Here's how the part is built. I have some questions about the finished solid (model axes, mm). A direction names the side the tool comes from. Coordinates: 2 decimals unless noted, no trailing zeros. Order: outer loops, then holes, each group sorted by start corner. A loop starts at its lowest first (then second) coordinate and runs counter-clockwise, first axis right, second up. Notation, with made-up numbers: M 36.25,41.5 L 93.25,41.5 A21 ccw 93.25,61.5 Z; hole C 11,18.5 d9. An arc over 180 degrees is marked long. One line per question, with ' | ' between items. Start each with the question number.
```python
from build123d import *

# Parameters (mm, degrees)
SKETCH1_W           = 100
SKETCH1_H           = 200
SKETCH1_W_2         = 67
SKETCH1_H_2         = 110
BOSS_EXTRUDE1_DEPTH = 2
SKETCH2_W           = 100
SKETCH2_H           = 200
SKETCH2_W_2         = 94
SKETCH2_H_2         = 194
BOSS_EXTRUDE2_DEPTH = 16.4
SKETCH3_R           = 1.15
BOSS_EXTRUDE3_DEPTH = 2
BOSS_EXTRUDE4_DEPTH = 25
SKETCH8_W           = 100
SKETCH8_H           = 110
BOSS_EXTRUDE5_DEPTH = 3
SKETCH9_W           = 11
SKETCH9_H           = 13
CUT_EXTRUDE2_DEPTH  = 36
SKETCH10_W          = 7
SKETCH10_H          = 3
CUT_EXTRUDE3_DEPTH  = 10
SKETCH11_W          = 3
SKETCH11_H          = 7
CUT_EXTRUDE4_DEPTH  = 10
SKETCH12_W          = 100
SKETCH12_H          = 17.4
CUT_EXTRUDE5_DEPTH  = 3
SKETCH13_W          = 146.237469439
SKETCH13_H          = 217.9364229
CUT_EXTRUDE6_DEPTH  = 57
SKETCH14_R          = 2
CUT_EXTRUDE7_DEPTH  = 57
SKETCH15_W          = 2
SKETCH15_H          = 10
SKETCH15_W_2        = 10
SKETCH15_H_2        = 2
BOSS_EXTRUDE6_DEPTH = 5
SKETCH16_W          = 10
SKETCH16_H          = 1.7
BOSS_EXTRUDE7_DEPTH = 2
SKETCH17_W          = 10
SKETCH17_H          = 1.7
BOSS_EXTRUDE8_DEPTH = 2


with BuildPart() as part:
    # Sketch1 → Boss-Extrude1 (new body)
    with BuildSketch(Plane(origin=(0, 0, 0), x_dir=(1, 0, 0), z_dir=(0, 1, 0))):
        Rectangle(SKETCH1_W, SKETCH1_H)
        with Locations((0, 35)):
            Rectangle(SKETCH1_W_2, SKETCH1_H_2, mode=Mode.SUBTRACT)
    extrude(amount=BOSS_EXTRUDE1_DEPTH)

    # Sketch2 → Boss-Extrude2 (add)
    with BuildSketch(Plane.XZ):
        Rectangle(SKETCH2_W, SKETCH2_H)
        Rectangle(SKETCH2_W_2, SKETCH2_H_2, mode=Mode.SUBTRACT)
    extrude(amount=BOSS_EXTRUDE2_DEPTH)

    # Sketch3 → Boss-Extrude3 (add)
    with BuildSketch(Plane.XZ.offset(16.4)):
        Polygon((-50, 100), (50, 100), (50, 10), (50, -9), (30, -9), (30, 1), (35, 1), (35, 10), (35, 80), (-35, 80), (-35, 10), (-35, 1), (-30, 1), (-30, -9), (-50, -9), (-50, 10), align=None)
        with Locations(Location((-35, 85, 0), (0, 0, 270))):
            Circle(SKETCH3_R, mode=Mode.SUBTRACT)
        with Locations(Location((35, 85, 0), (0, 0, 270))):
            Circle(SKETCH3_R, mode=Mode.SUBTRACT)
        with Locations(Location((-35, -4, 0), (0, 0, 270))):
            Circle(SKETCH3_R, mode=Mode.SUBTRACT)
        with Locations(Location((35, -4, 0), (0, 0, 270))):
            Circle(SKETCH3_R, mode=Mode.SUBTRACT)
    extrude(amount=BOSS_EXTRUDE3_DEPTH)

    # Sketch5 → Boss-Extrude4 (add)
    with BuildSketch(Plane.XZ.offset(16.4)):
        Polygon((-50, -100), (50, -100), (50, -97), (50, 10), (47, 10), (47, -97), (-47, -97), (-47, 10), (-50, 10), (-50, -97), align=None)
    extrude(amount=BOSS_EXTRUDE4_DEPTH)

    # Sketch8 → Boss-Extrude5 (add)
    with BuildSketch(Plane.XZ.offset(41.4)):
        with Locations((0, -45)):
            Rectangle(SKETCH8_W, SKETCH8_H)
    extrude(amount=BOSS_EXTRUDE5_DEPTH)

    # Sketch9 → Cut-Extrude2 (cut)
    with BuildSketch(Plane(origin=(0, -16.4, 0), x_dir=(1, 0, 0), z_dir=(0, 1, 0))):
        with Locations((-28.65, -74.5)):
            Rectangle(SKETCH9_W, SKETCH9_H)
        with Locations((-0.71, -74.5)):
            Rectangle(SKETCH9_W, SKETCH9_H)
        with Locations((24.69, -74.5)):
            Rectangle(SKETCH9_W, SKETCH9_H)
        with Locations((-28.65, -49.1)):
            Rectangle(SKETCH9_W, SKETCH9_H)
        with Locations((-0.71, -49.1)):
            Rectangle(SKETCH9_W, SKETCH9_H)
        with Locations((24.69, -49.1)):
            Rectangle(SKETCH9_W, SKETCH9_H)
    extrude(amount=CUT_EXTRUDE2_DEPTH, mode=Mode.SUBTRACT)

    # Sketch10 → Cut-Extrude3 (cut)
    with BuildSketch(Plane.XZ.offset(44.4)):
        with Locations((-39.5, 5)):
            Rectangle(SKETCH10_W, SKETCH10_H)
        with Locations((39.5, 5)):
            Rectangle(SKETCH10_W, SKETCH10_H)
    extrude(amount=-CUT_EXTRUDE3_DEPTH, mode=Mode.SUBTRACT)

    # Sketch11 → Cut-Extrude4 (cut)
    with BuildSketch(Plane.XZ.offset(18.4)):
        with Locations((-45, 91.5)):
            Rectangle(SKETCH11_W, SKETCH11_H)
        with Locations((45, 91.5)):
            Rectangle(SKETCH11_W, SKETCH11_H)
    extrude(amount=-CUT_EXTRUDE4_DEPTH, mode=Mode.SUBTRACT)

    # Sketch12 → Cut-Extrude5 (cut)
    with BuildSketch(Plane.XY.offset(100)):
        with Locations((0, -9.7)):
            Rectangle(SKETCH12_W, SKETCH12_H)
    extrude(amount=-CUT_EXTRUDE5_DEPTH, mode=Mode.SUBTRACT)

    # Sketch13 → Cut-Extrude6 (cut)
    with BuildSketch(Plane.XZ):
        with Locations((11.358250054, -1.301466152)):
            Rectangle(SKETCH13_W, SKETCH13_H)
    extrude(amount=CUT_EXTRUDE6_DEPTH, mode=Mode.SUBTRACT)

    # Sketch14 → Cut-Extrude7 (cut)
    with BuildSketch(Plane(origin=(0, 2, 0), x_dir=(1, 0, 0), z_dir=(0, 1, 0))):
        with Locations(Location((-41, -91, 0), (0, 0, 270))):
            Circle(SKETCH14_R)
        with Locations(Location((41, -91, 0), (0, 0, 270))):
            Circle(SKETCH14_R)
        with Locations(Location((41, -32.5, 0), (0, 0, 270))):
            Circle(SKETCH14_R)
        with Locations(Location((-41, -32.5, 0), (0, 0, 270))):
            Circle(SKETCH14_R)
        with Locations(Location((-41, 91, 0), (0, 0, 270))):
            Circle(SKETCH14_R)
        with Locations(Location((41, 91, 0), (0, 0, 270))):
            Circle(SKETCH14_R)
    extrude(amount=-CUT_EXTRUDE7_DEPTH, mode=Mode.SUBTRACT)

    # Sketch15 → Boss-Extrude6 (add)
    with BuildSketch(Plane.XZ):
        with Locations((-36.8, 3.147463841)):
            Rectangle(SKETCH15_W, SKETCH15_H)
        with Locations((-36.8, -72.12250392)):
            Rectangle(SKETCH15_W, SKETCH15_H)
        with Locations((40.8, 5)):
            Rectangle(SKETCH15_W, SKETCH15_H)
        with Locations((40.8, -72.12250392)):
            Rectangle(SKETCH15_W, SKETCH15_H)
        with Locations((-1.11415266, -96)):
            Rectangle(SKETCH15_W_2, SKETCH15_H_2)
        with Locations((-1.11415266, 27)):
            Rectangle(SKETCH15_W_2, SKETCH15_H_2)
    extrude(amount=BOSS_EXTRUDE6_DEPTH)

    # Sketch16 → Boss-Extrude7 (add)
    with BuildSketch(Plane(origin=(-35.8, 0, 0), x_dir=(0, 0, -1), z_dir=(1, 0, 0))):
        with Locations((-3.147463841, -4.15)):
            Rectangle(SKETCH16_W, SKETCH16_H)
        with Locations((72.12250392, -4.15)):
            Rectangle(SKETCH16_W, SKETCH16_H)
    extrude(amount=BOSS_EXTRUDE7_DEPTH)

    # Sketch17 → Boss-Extrude8 (add)
    with BuildSketch(Plane.ZY.offset(-39.8)):
        with Locations((5, -4.15)):
            Rectangle(SKETCH17_W, SKETCH17_H)
        with Locations((-72.12250392, -4.15)):
            Rectangle(SKETCH17_W, SKETCH17_H)
    extrude(amount=BOSS_EXTRUDE8_DEPTH)


solid = part.part
```
1. Which directions (+Z, -Z, +X, -X, +Y, -Y) give clear straight access to the entire face, cutting with the end or side of a thin tool? Please do faces 1 (the face through (40, -3, -67.123)), 2 (the face through (41.8, -2, 5)), 3 (the face through (-36, -3, -77.123)).
2. Will these pins go through, and if not, where does the flat tip stop? pin 1 (4 mm diameter, centred on y = -3.5, z = -71, fed in from +X); pin 2 (2.5 mm diameter, centred on y = -2.5, z = 7.5, fed in from -X); pin 3 (1.6 mm diameter, centred on y = -2.5, z = -96.5, fed in from +X).
3. We'd pull the mould along Z, two halves only. Please class faces 4 (the face through (-36, -3, -1.853)), 5 (the face through (-37.8, -2, 3)), 6 (the face through (-1, -2, 28)): released by +Z, released by -Z, zero draft, split by the parting line, or undercut.
4. Imagine slicing it at D-D (y = -2). List the corners of the cut face in (x, z) for me, then the cut area to 3 significant figures.
5. Imagine slicing it at C-C (z = 91). List the corners of the cut face in (x, y) for me, then the cut area to 3 significant figures.
6. Imagine slicing it at B-B (z = 3.5). List the corners of the cut face in (x, y) for me.
7. Imagine slicing it at A-A (x = -41). List the corners of the cut face in (y, z) for me.
8. I need wall thicknesses on line 1 (X direction, y = 1.05, z = 91); line 2 (Z direction, x = -6, y = 1.25); line 3 (Z direction, x = -16, y = 1.25). Which ranges of each line are inside material? Lowest first, please.
Entries:
1) face 1: +X, -X, -Y | face 2: +Z, -Z, +X, -Y | face 3: -Z, +X, -X, -Y
2) pin 1: x = 41.8 | pin 2: x = -37.8 | pin 3: x = 3.89
3) face 4: undercut | face 5: zero draft | face 6: released by +Z
4) outline: M -37.8,-77.12 L -35.8,-77.12 L -35.8,-67.12 L -37.8,-67.12 Z; M -37.8,-1.85 L -35.8,-1.85 L -35.8,8.15 L -37.8,8.15 Z; M -6.11,-97 L 3.89,-97 L 3.89,-95 L -6.11,-95 Z; M -6.11,26 L 3.89,26 L 3.89,28 L -6.11,28 Z; M 39.8,-77.12 L 41.8,-77.12 L 41.8,-67.12 L 39.8,-67.12 Z; M 39.8,0 L 41.8,0 L 41.8,10 L 39.8,10 Z | area: 120 mm²
5) outline: M -50,0 L -43,0 L -43,2 L -50,2 Z; M -39,0 L 39,0 L 39,2 L -39,2 Z; M 43,0 L 50,0 L 50,2 L 43,2 Z | area: 184 mm²
6) outline: M -50,0 L -37.8,0 L -37.8,-5 L -33.8,-5 L -33.8,-3.3 L -35.8,-3.3 L -35.8,0 L -33.5,0 L -33.5,2 L -50,2 Z; M 33.5,0 L 39.8,0 L 39.8,-3.3 L 37.8,-3.3 L 37.8,-5 L 41.8,-5 L 41.8,0 L 50,0 L 50,2 L 33.5,2 Z
7) outline: M 0,-100 L 2,-100 L 2,-93 L 0,-93 Z; M 0,-89 L 2,-89 L 2,30.5 L 0,30.5 Z; M 0,34.5 L 2,34.5 L 2,89 L 0,89 Z; M 0,93 L 2,93 L 2,100 L 0,100 Z
8) line 1: -50 to -43, -39 to 39, 43 to 50 | line 2: -100 to -90, 20 to 42.6, 55.6 to 68, 81 to 100 | line 3: -100 to -90, 20 to 100
